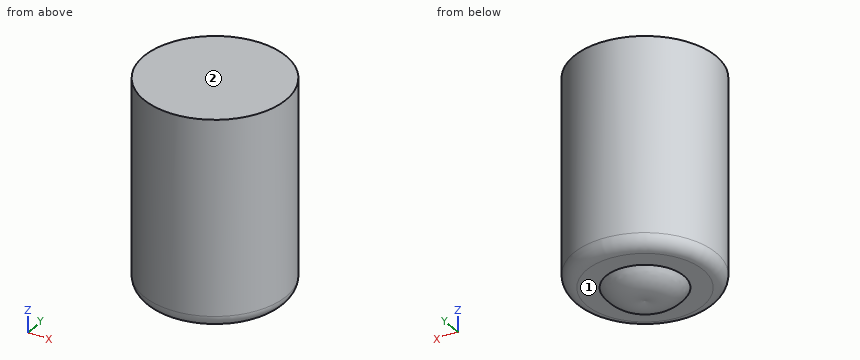
```python
from build123d import *

# Parameters (mm, degrees)
F0_R     = 5.5
F1_DEPTH = 16
F2_R     = 1
F3_T     = -1.5


with BuildPart() as f1:
    # F0 (on Top) → F1 (new body)
    with BuildSketch(Plane.XY):
        Circle(F0_R)
    extrude(amount=-F1_DEPTH)

    # F2
    f2_edges = [f1.edges().sort_by_distance(p)[0] for p in [
        (-5.5, 0, -16),
    ]]
    fillet(f2_edges, radius=F2_R)

    # F3 (hollow: no face is removed)
    offset(amount=F3_T, mode=Mode.SUBTRACT)

    # F4 (on Front) → F5 (revolve)
    with BuildSketch(Plane.XZ):
        with BuildLine():
            Line((3, -16), (0, -16))
            Line((0, -16), (0, -17))
            ThreePointArc((0, -17), (1.6716371784, -17.0149115353), (3, -16))
        make_face()
    revolve(axis=Axis((0, 0, -16.5), (0, 0, -1)))


solid = f1.part
```
Input: part model. Units: mm. Frame: model coordinates. Face numbers are marked on the shaded views. A direction names the side the tool comes from. Round coordinates to 2 decimals unless told otherwise and drop trailing zeros. Write each loop counter-clockwise with the first axis right and the second up, starting at its lowest first coordinate (ties: lowest second). Pieces come first, ordered by that corner, then holes. Notation, with made-up numbers: M 17.5,-25 L 68.5,-25 A10 ccw 68.5,-14 Z; hole C -21.75,77 d5. An arc over 180 degrees is marked long. Write each question's results on one line, items separated by ' | '.
Q1. Pin query (flat end, axial travel): P1, Ø1.5, axis at y = -3.5, z = -6.5, coming from the +X side; P2, Ø2.5, axis at x = 1.5, y = 0.5, coming from the -Z side; P3, Ø3, axis at y = -4, z = -4, coming from the -X side; P4, Ø6, axis at x = -4, z = -15, coming from the +Y side. Return the tip coordinate at first contact, or that it passes through.
Results:
P1: stops at x = 4.76 | P2: stops at z = -17.15 | P3: stops at x = -4.9 | P4: stops at y = 5.41
Q2. Access query for the marked faces 1 and 2. Directions: +Z, -Z, +X, -X, +Y, -Y. A direction counts if a zero-diameter tool reaches every point of the face in a straight line with its end or side. Return the directions, or none.
Results:
face 1: -Z | face 2: +Z, +X, -X, +Y, -Y
Q3. Section query A-A (z = -9.75). Return loops of the section in (x, y).
Results:
outline: C 0,0 d11; hole C 0,0 d8
Q4. Line query: line 1 along Z through (x, y) = (0.5, -3.25); line 2 along Y through (x, z) = (0, -6.5); line 3 along Y through (x, z) = (-3, -11). Output: solid intervals per line, ascending.
Results:
line 1: z = -16 to -14.5, -1.5 to 0 | line 2: y = -5.5 to -4, 4 to 5.5 | line 3: y = -4.61 to -2.65, 2.65 to 4.61
Q5. Section query B-B (z = -15.25). Return loops of the section in (x, y).
Results:
outline: C 0,0 d10.94
